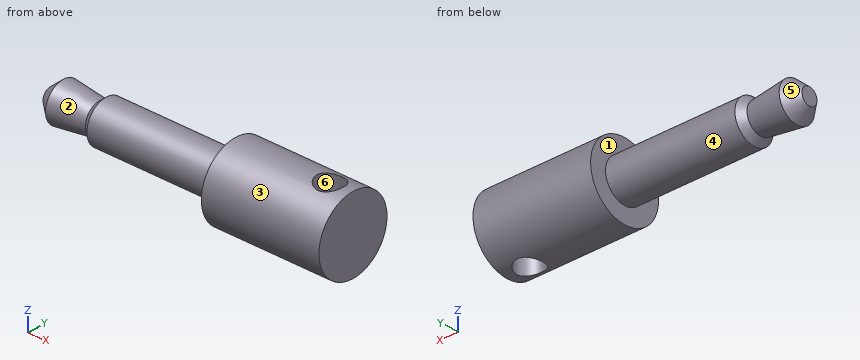
Autodesk Inventor part; units mm, degrees
ref_plane "YZ Plane" through (0, 0, 0) normal (1, 0, 0) x (0, 1, 0)
ref_plane "XZ Plane" through (0, 0, 0) normal (0, 1, 0) x (-1, 0, 0)
ref_plane "XY Plane" through (0, 0, 0) normal (0, 0, 1) x (1, 0, 0)
sketch "Sketch1" plane through (0, 0, 0) normal (0, 0, 1) x (1, 0, 0)
  line L0 (0, 0) -> (25.9627, 0)
  line L1 (0, 0) -> (0, 0.495)
  line L2 (0, 0.495) -> (0.75, 1.155)
  line L3 (0.75, 1.155) -> (2.9, 0.9)
  line L4 (2.9, 0.9) -> (3.3, 1.25)
  line L5 (3.3, 1.25) -> (11, 1.25)
  line L6 (11, 1.25) -> (11, 0)
  line L7 (11, 0) -> (0, 0)
  dimension "d0" = 0.99
  dimension "d1" = 2.5
  dimension "d2" = 2.31
  dimension "d3" = 0.75
  dimension "d4" = 1.8
  dimension "d5" = 2.9
  dimension "d6" = 3.3
  dimension "d7" = 11
revolve "Revolution1" add sketch "Sketch1" angle 360 about axis through (0, 0, 0) along (1, 0, 0)
sketch "Sketch2" plane through (11, 0, 0) normal (1, 0, 0) x (0, 0, -1)
  circle A0 centre (0, 0) radius 1.25
  circle A1 centre (0, 0) radius 2.225
  dimension "d9" = 4.45
extrude "Extrusion1" add sketch "Sketch2" along normal blind 7 contours A0 | A1
sketch "Sketch3" plane through (0, 0, 0) normal (0, 0, 1) x (1, 0, 0)
  circle A0 centre (16.6444, 0) radius 0.7937
  line L0 (18, 2.225) -> (18, -2.225)
  point P0 (0, 0)
  dimension "d12" = 1.5875
  dimension "d13" = 1.3556
extrude "Extrusion2" cut sketch "Sketch3" along normal through all both and the other way through all
properties part number "safe_rbf"
For this review, take the finished solid that the model builds, in its own axes (mm). Face numbers are marked on the shaded views. A direction names the side the tool comes from. Round coordinates to 2 decimals unless told otherwise and drop trailing zeros. Write each loop counter-clockwise with the first axis right and the second up, starting at its lowest first coordinate (ties: lowest second). Pieces come first, ordered by that corner, then holes. Notation, with made-up numbers: (-10, -22.75) -> (19, -22.75) arc R23 ccw to (19, -4.75) -> close; hole circle Ø3 at (89, 9). An arc over 180 degrees is marked (long way). Use one line per item in the form item = value.
Q1. Consider section C-C (x = 3.5). State the section outline as (y, z) points, then the cut area to 3 significant figures.
Resolved:
outline = circle Ø2.5 at (0, 0)
area = 4.91 mm²
Q2. Consider section D-D (y = -1.9). State the section outline as (x, z) points.
Resolved:
outline = (11, -1.16) -> (18, -1.16) -> (18, 1.16) -> (11, 1.16) -> close
Q3. The part is to be moulded in two halves that separate along X. For the marked faces 4, 5 and 6, say which applies: released by +X, released by -X, zero draft, split by the parting line, or undercut.
Resolved:
face_4 = zero draft
face_5 = released by -X
face_6 = undercut
Q4. Machinability: for the marked faces 1, 2 and 3, which of the approach directions +Z, -Z, +X, -X, +Y, -Y give a long, thin tool a straight path to every point of the face, cutting with its end or side? Answer none if there is none.
Resolved:
face_1 = -X
face_2 = none
face_3 = +X, -X
Q5. To check wall thickness, follow probe 1 along X at (y, z) = (0, -0.25); probe 2 along Z at (x, y) = (5.75, -0.05); probe 3 along X at (y, z) = (0, 1.2). State the ranges of each line that lie inside material, in increasing order. Write a range as from..to.
Resolved:
probe_1 = 0..15.85, 17.44..18
probe_2 = -1.25..1.25
probe_3 = 3.24..15.85, 17.44..18
Q6. Consider section A-A (z = 0). State the section outline as (x, y) points (3 decimals).
Resolved:
outline = (0, -0.495) -> (0.75, -1.155) -> (2.9, -0.9) -> (3.3, -1.25) -> (11, -1.25) -> (11, -2.225) -> (18, -2.225) -> (18, 2.225) -> (11, 2.225) -> (11, 1.25) -> (3.3, 1.25) -> (2.9, 0.9) -> (0.75, 1.155) -> (0, 0.495) -> close; hole circle Ø1.587 at (16.644, 0)
Q7. Clearance check with flat-ended pins moving along their axes: pin 1 Ø1.5 at (x, y) = (11.5, 0.5) entering from -Z (3 decimals); pin 2 Ø2 at (x, z) = (3, -1.5) entering from +Y; pin 3 Ø2 at (x, y) = (6, -0.5) entering from -Z; pin 4 Ø1 at (x, y) = (16.64, 0) entering from -Z. State where each tip first meets the part, or that it passes through.
Resolved:
pin_1 = -2.225
pin_2 = 1.12
pin_3 = -1.25
pin_4 = through
Q8. Consider section B-B (y = 0). State the section outline as (x, z) points (3 decimals), then the cut area to 3 significant figures.
Resolved:
outline = (0, -0.495) -> (0.75, -1.155) -> (2.9, -0.9) -> (3.3, -1.25) -> (11, -1.25) -> (11, -2.225) -> (15.851, -2.225) -> (15.851, 2.225) -> (11, 2.225) -> (11, 1.25) -> (3.3, 1.25) -> (2.9, 0.9) -> (0.75, 1.155) -> (0, 0.495) -> close; (17.438, -2.225) -> (18, -2.225) -> (18, 2.225) -> (17.438, 2.225) -> close
area = 49.9 mm²
